Work out the finished part from the listing and answer in its coordinate system (mm). Face numbers are marked on the shaded views. A direction names the side the tool comes from. Coordinates: 2 decimals unless noted, no trailing zeros. Loops run counter-clockwise (first coordinate to the right, second up) from the corner with the lowest first, then second, coordinate; pieces in that order, holes last. Notation, with made-up numbers: (7.25, 44) - (43.25, 44) arc R32 cw to (43.25, 75) - close; hole circle Ø10 at (-19, -30). An arc over 180 degrees is marked (long way). Write each question's results on one line, items separated by ' | '. Start each with the question number.
Item 1: Section A-A, the plane z = 46 is taken. Write down the section's boundary in (x, y), plus the area to 3 significant figures.
Item 2: A tool of negligible diameter and unlimited length cuts with its end or side. For the marked faces 1 and 2, from which of +Z, -Z, +X, -X, +Y, -Y can it reach the whole face along a straight path? Write none if from no direction.
Item 3: Section B-B, the plane x = 51 is taken. Write down the section's boundary in (y, z).
Item 4: Section C-C, the plane y = 39.5 is taken. Write down the section's boundary in (x, z).
Item 5: Each of these flat-tipped pins is pushed along its axis until it touches: pin 1 Ø1.5 at (x, z) = (-37, 42.5) entering from -Y; pin 2 Ø8 at (x, y) = (24, 50) entering from -Z. Where does it stop, or does it pass through?
Item 6: Consider probe 1 along X at (y, z) = (37, 33); probe 2 along Y at (x, z) = (-30, 48). Determine where each line is inside the solid, lowest interval first. Write a range as [from, to].
from build123d import *

# Parameters (mm, degrees)
F0_W     = 39.715842
F0_H     = 25.4
F1_DEPTH = 25.4
F2_DEPTH = 25.4


with BuildPart() as f1:
    # F0 (on Top) → F1 (new body)
    with BuildSketch(Plane.XY):
        Polygon((23.808891, 69.293525), (-88.875267, 69.293525), (-88.875267, -6.906475), (-38.075267, -6.906475), (-38.075267, 43.893525), (23.808891, 43.893525), align=None)
        with Locations((43.666812, 56.593525)):
            Rectangle(F0_W, F0_H)
    extrude(amount=F1_DEPTH)

    # F1_face (on face) → F2 (join)
    with BuildSketch(Plane(origin=(-32.995267, 41.353525, 25.4), x_dir=(1, 0, 0), z_dir=(0, 0, 1))):
        Polygon((96.52, 27.94), (-55.88, 27.94), (-55.88, -48.26), (-5.08, -48.26), (-5.08, 2.54), (96.52, 2.54), align=None)
    extrude(amount=F2_DEPTH)


solid = f1.part
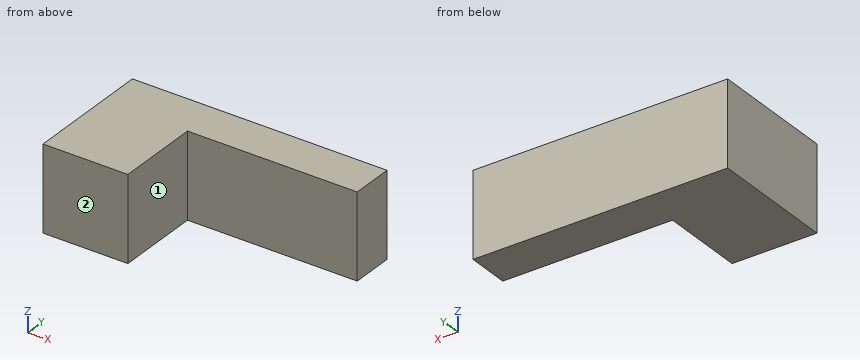
Answer key:
1) outline: (-88.88, -6.91) - (-38.08, -6.91) - (-38.08, 43.89) - (63.52, 43.89) - (63.52, 69.29) - (-88.88, 69.29) - close | area: 6,450 mm^2
2) face 1: +Z, -Z, +X, -Y | face 2: +Z, -Z, +X, -X, -Y
3) outline: (43.89, 0) - (69.29, 0) - (69.29, 50.8) - (43.89, 50.8) - close
4) outline: (-88.88, 0) - (-38.08, 0) - (-38.08, 50.8) - (-88.88, 50.8) - close
5) pin 1: stops at y = 43.89 | pin 2: stops at z = 0
6) probe 1: x = [-88.88, -38.08] | probe 2: y = [43.89, 69.29]
